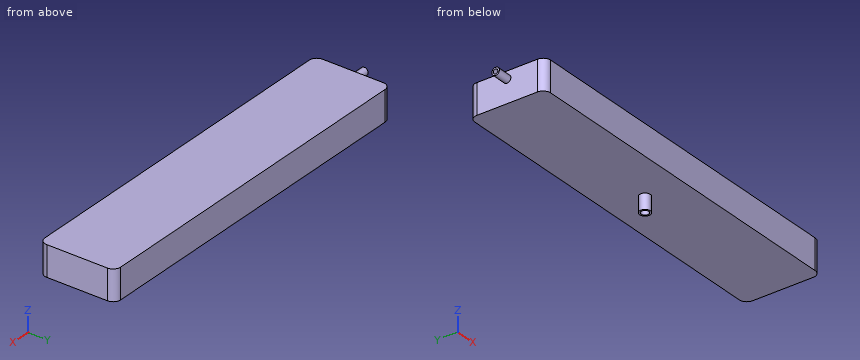
```python
from build123d import *

# Parameters (mm, degrees)
F0_W     = 240
F0_H     = 50
F0_R     = 3.5
F1_DEPTH = 20
F2_R     = 5
F4_R     = 3.5
F4_R_2   = 2.5
F5_DEPTH = 10
F3_R     = 2.5
F3_R_2   = 1.5
F6_DEPTH = 10


with BuildPart() as f1:
    # F0 (on Top) → F1 (new body)
    with BuildSketch(Plane.XY):
        Rectangle(F0_W, F0_H)
        Circle(F0_R, mode=Mode.SUBTRACT)
        Circle(F0_R)
    extrude(amount=F1_DEPTH)

    # F2
    f2_edges = [f1.edges().sort_by_distance(p)[0] for p in [
        (-120, -25, 10),
        (120, -25, 10),
        (120, 25, 10),
        (-120, 25, 10),
    ]]
    fillet(f2_edges, radius=F2_R)

    # F4 (on face) → F5 (join)
    with BuildSketch(Plane(origin=(0, 0, 0), x_dir=(1, 0, 0), z_dir=(0, 0, -1))):
        Circle(F4_R)
        Circle(F4_R_2, mode=Mode.SUBTRACT)
    extrude(amount=F5_DEPTH)

    # F3 (on face) → F6 (join)
    with BuildSketch(Plane(origin=(-120, 0, 0), x_dir=(0, -1, 0), z_dir=(-1, 0, 0))):
        with Locations((0, 15)):
            Circle(F3_R)
        with Locations((0, 15)):
            Circle(F3_R_2, mode=Mode.SUBTRACT)
    extrude(amount=F6_DEPTH)


solid = f1.part
```
Could you check a few things on this model? Use its own coordinates, in mm. Coordinates: 2 decimals unless noted, no trailing zeros. Write each loop counter-clockwise with the first axis right and the second up, starting at its lowest first coordinate (ties: lowest second). Pieces come first, ordered by that corner, then holes. Notation, with made-up numbers: (81, 26) -> (102, 26) arc R19 ccw to (102, 55) -> close; hole circle Ø9 at (1, 40). An arc over 180 degrees is marked (long way). Write item = value, one per line. Start each with the question number.
(1) Will these pins go through, and if not, where does the flat tip stop? pin 1 (12 mm diameter, centred on x = -83, y = -3, fed in from -Z); pin 2 (6 mm diameter, centred on y = -2, z = 6, fed in from -X).
(2) I want a section at B-B (x = 0). Please give me the cut outline in (y, z).
(3) I want a section at A-A (z = 6.25). Please give me the cut outline in (x, y).
(4) I want a section at D-D (y = -15). Please give me the cut outline in (x, z).
(5) I want a section at C-C (z = -7). Please give me the cut outline in (x, y), plus the area to 3 significant figures.
(6) I need wall thicknesses on line 1 (Y direction, x = 0, z = -5); line 2 (Z direction, x = -117.5, y = -2.5). Which ranges of each line are inside material? Lowest first, please. Write a range as [from, to].
Result set:
q1.pin_1 = 0
q1.pin_2 = -120
q2.outline = (-25, 0) -> (-3.5, 0) -> (-3.5, -10) -> (-2.5, -10) -> (-2.5, 0) -> (2.5, 0) -> (2.5, -10) -> (3.5, -10) -> (3.5, 0) -> (25, 0) -> (25, 20) -> (-25, 20) -> close
q3.outline = (-120, -20) arc R5 ccw to (-115, -25) -> (115, -25) arc R5 ccw to (120, -20) -> (120, 20) arc R5 ccw to (115, 25) -> (-115, 25) arc R5 ccw to (-120, 20) -> close
q4.outline = (-120, 0) -> (120, 0) -> (120, 20) -> (-120, 20) -> close
q5.outline = circle Ø7 at (0, 0); hole circle Ø5 at (0, 0)
q5.area = 18.8 mm2
q6.line_1 = [-3.5, -2.5], [2.5, 3.5]
q6.line_2 = [0, 20]
